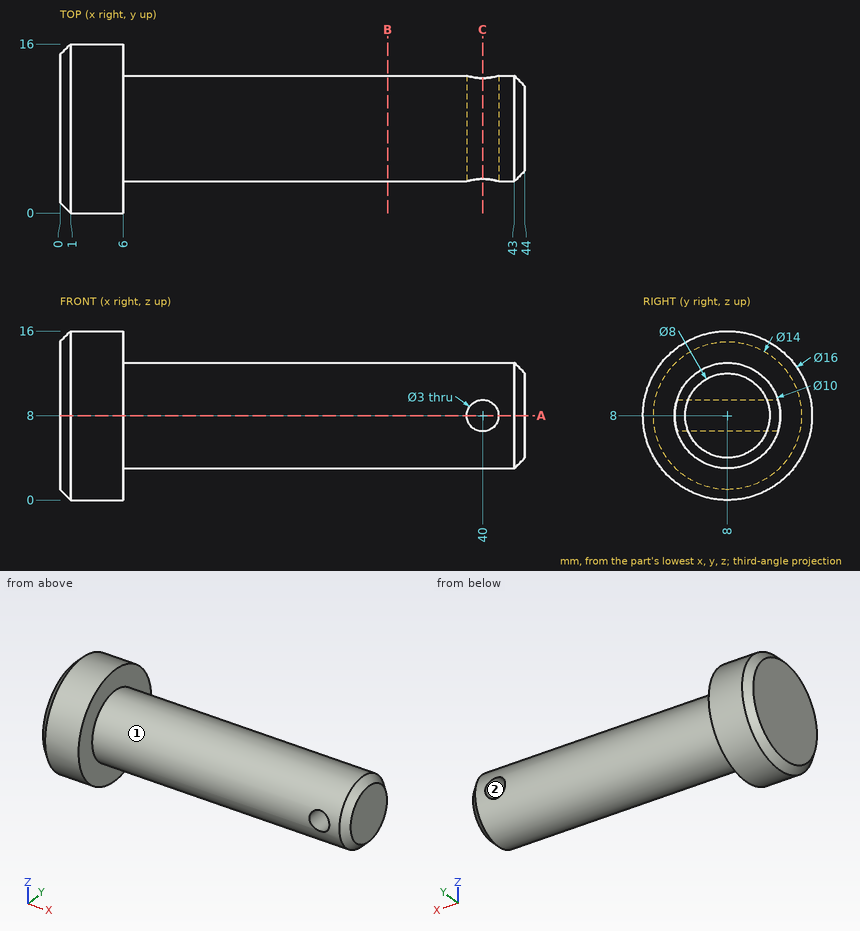
Design review of the part shown in the three views and the two pictorial views. Dimensions are in mm from the part's minimum x, y and z. A direction names the side the tool comes from. Give positions to 0.01 mm unless a question says otherwise; leave off trailing zeros. Write each loop counter-clockwise with the first axis right and the second up, starting at its lowest first coordinate (ties: lowest second). Pieces come first, ordered by that corner, then holes.
(1) Clearance check with flat-ended pins moving along their axes: pin 1 Ø6 at (x, z) = (24.5, 7) entering from +Y; pin 2 Ø2 at (x, y) = (19.5, 12.5) entering from +Z; pin 3 Ø8 at (x, z) = (12.5, 6) entering from -Y. State where each tip first meets the part, or that it passes through.
Checked values:
pin 1: stops at y = 13
pin 2: stops at z = 11.57
pin 3: stops at y = 3
(2) Tool access review of the marked faces 1 and 2: name each direction out of +Z, -Z, +X, -X, +Y, -Y from which nothing blocks a thin tool from reaching the whole face with its end or side.
Checked values:
face 1: +X
face 2: +Y, -Y
(3) Add section C-C (x = 40). Give the boundary of the cut face in (y, z).
Checked values:
outline: (3.23, 6.5) arc R5 ccw to (12.77, 6.5) - close; (3.23, 9.5) - (12.77, 9.5) arc R5 ccw to start
(4) Add section B-B (x = 31). Give the boundary of the cut face in (y, z).
Checked values:
outline: circle Ø10 at (8, 8)
(5) Add section A-A (z = 8). Give the boundary of the cut face in (x, y), and give its area (3 significant figures).
Checked values:
outline: (0, 1) - (1, 0) - (6, 0) - (6, 3) - (38.5, 3) - (38.5, 13) - (6, 13) - (6, 16) - (1, 16) - (0, 15) - close; (41.5, 3) - (43, 3) - (44, 4) - (44, 12) - (43, 13) - (41.5, 13) - close
area: 444 mm2
(6) Wall thickness on line 1 along Z through (x, y) = (40, 5); line 2 along X through (y, z) = (8.25, 8); line 3 along Z through (x, y) = (25.5, 11): over which ranges is each line inside the solid? List them lowest first.
Checked values:
line 1: z = 4 to 6.5, 9.5 to 12
line 2: x = 0 to 38.5, 41.5 to 44
line 3: z = 4 to 12
